The listing builds one solid part. Answer for the finished solid, in the listing's coordinates (mm). A direction names the side the tool comes from. Round coordinates to 2 decimals unless told otherwise and drop trailing zeros. Write each loop counter-clockwise with the first axis right and the second up, starting at its lowest first coordinate (ties: lowest second). Pieces come first, ordered by that corner, then holes.
Item 1: For a pull along X with two mould halves and no side action, classify faces 3 (the face through (49.756, 75.175, 14.79)), 4 (the face through (74.931, -1, 15)), 5 (the face through (-67, 0, 0)) as +X half, -X half, draft (parallel to the pull), parting line (faces both ways), or undercut.
Item 2: Find section A-A on y = -25.5. Give the vertices of the cut face in (x, z), then the cut area to 3 significant figures.
Item 3: Find the intervals of material crossed by probe 1 along X at (y, z) = (-40, 11.5); probe 2 along Y at (x, z) = (-3, 15.5); probe 3 along Y at (x, z) = (-54.5, 23.5), in increasing order.
Item 4: Find section C-C on z = 15.75. Give the vertices of the cut face in (x, y).
Item 5: A tool of negligible diameter and unlimited length cuts with its end or side. For faces 1 (the face through (-49.89, -75.18, 14.79)), 2 (the face through (-75.069, -1, 15)), from which of +Z, -Z, +X, -X, +Y, -Y can it reach the whole face along a straight path? Write none if from no direction.
Item 6: Find section B-B on x = 31. Give the vertices of the cut face in (y, z), then the cut area to 3 significant figures.
Item 7: Find section D-D on y = 81.25. Give the vertices of the cut face in (x, z).
```python
from build123d import *

# Parameters (mm, degrees)
F0_W     = 150
F0_H     = 200
F0_W_2   = 137.5
F0_H_2   = 187.5
F0_R     = 5
F0_R_2   = 2.5
F1_DEPTH = 30


with BuildPart() as f1:
    # F0 (on Top) → F1 (new body)
    with BuildSketch(Plane.XY):
        with Locations((-0.0686573694, 0)):
            Rectangle(F0_W, F0_H)
        with Locations((-0.0686573694, 0)):
            Rectangle(F0_W_2, F0_H_2, mode=Mode.SUBTRACT)
        with Locations((-0.0686573694, 0)):
            Rectangle(F0_W_2, F0_H_2)
        Polygon((-62.5686573694, 62.5), (-62.5686573694, 87.5), (-37.5686573694, 87.5), (37.4313426306, 87.5), (62.4313426306, 87.5), (62.4313426306, 62.5), (62.4313426306, -62.5), (62.4313426306, -87.5), (37.4313426306, -87.5), (-37.5686573694, -87.5), (-62.5686573694, -87.5), (-62.5686573694, -62.5), align=None, mode=Mode.SUBTRACT)
        Polygon((-37.5686573694, 87.5), (-62.5686573694, 87.5), (-62.5686573694, 62.5), align=None)
        with Locations((-56.3186573694, 81.25)):
            Circle(F0_R, mode=Mode.SUBTRACT)
        Polygon((62.4313426306, 87.5), (37.4313426306, 87.5), (62.4313426306, 62.5), align=None)
        with Locations((56.1813426306, 81.25)):
            Circle(F0_R, mode=Mode.SUBTRACT)
        Polygon((62.4313426306, -87.5), (62.4313426306, -62.5), (37.4313426306, -87.5), align=None)
        with Locations((56.1813426306, -81.25)):
            Circle(F0_R, mode=Mode.SUBTRACT)
        Polygon((-37.5686573694, -87.5), (-62.5686573694, -62.5), (-62.5686573694, -87.5), align=None)
        with Locations((-56.3186573694, -81.25)):
            Circle(F0_R, mode=Mode.SUBTRACT)
        with Locations((-56.3186573694, 81.25)):
            Circle(F0_R)
        with Locations((-56.3186573694, 81.25)):
            Circle(F0_R_2, mode=Mode.SUBTRACT)
        with Locations((56.1813426306, 81.25)):
            Circle(F0_R)
        with Locations((56.1813426306, 81.25)):
            Circle(F0_R_2, mode=Mode.SUBTRACT)
        with Locations((56.1813426306, -81.25)):
            Circle(F0_R)
        with Locations((56.1813426306, -81.25)):
            Circle(F0_R_2, mode=Mode.SUBTRACT)
        with Locations((-56.3186573694, -81.25)):
            Circle(F0_R)
        with Locations((-56.3186573694, -81.25)):
            Circle(F0_R_2, mode=Mode.SUBTRACT)
    extrude(amount=F1_DEPTH)


solid = f1.part
```
Check values:
1. face 3: undercut
1. face 4: +X half
1. face 5: draft
2. outline: (-75.07, 0) - (-62.57, 0) - (-62.57, 30) - (-75.07, 30) - close; (62.43, 0) - (74.93, 0) - (74.93, 30) - (62.43, 30) - close
2. area: 750 mm2
3. probe 1: x = -75.07 to -62.57, 62.43 to 74.93
3. probe 2: y = -100 to -87.5, 87.5 to 100
3. probe 3: y = -100 to -82.97, -79.53 to -70.57, 70.57 to 79.53, 82.97 to 100
4. outline: (-75.07, -100) - (74.93, -100) - (74.93, 100) - (-75.07, 100) - close; hole (-62.57, -62.5) - (-37.57, -87.5) - (37.43, -87.5) - (62.43, -62.5) - (62.43, 62.5) - (37.43, 87.5) - (-37.57, 87.5) - (-62.57, 62.5) - close; hole circle Ø5 at (-56.32, -81.25); hole circle Ø5 at (-56.32, 81.25); hole circle Ø5 at (56.18, -81.25); hole circle Ø5 at (56.18, 81.25)
5. face 1: +Z, -Z
5. face 2: +Z, -Z, -X, +Y, -Y
6. outline: (-100, 0) - (-87.5, 0) - (-87.5, 30) - (-100, 30) - close; (87.5, 0) - (100, 0) - (100, 30) - (87.5, 30) - close
6. area: 750 mm2
7. outline: (-75.07, 0) - (-58.82, 0) - (-58.82, 30) - (-75.07, 30) - close; (-53.82, 0) - (-43.82, 0) - (-43.82, 30) - (-53.82, 30) - close; (43.68, 0) - (53.68, 0) - (53.68, 30) - (43.68, 30) - close; (58.68, 0) - (74.93, 0) - (74.93, 30) - (58.68, 30) - close
